from build123d import *

# Parameters (mm, degrees)
SKETCH1_W           = 69.3
SKETCH1_H           = 27
BOSS_EXTRUDE1_DEPTH = 13.2
SKETCH2_R           = 4.55
BOSS_EXTRUDE2_DEPTH = 2.25
SKETCH3_R           = 3.1
BOSS_EXTRUDE3_DEPTH = 6.25
SKETCH4_W           = 4.5
SKETCH4_H           = 12
BOSS_EXTRUDE4_DEPTH = 14


with BuildPart() as part:
    # Sketch1 → Boss-Extrude1 (new body)
    with BuildSketch(Plane.XY):
        with Locations((-34.65, 13.5)):
            Rectangle(SKETCH1_W, SKETCH1_H)
    extrude(amount=BOSS_EXTRUDE1_DEPTH)

    # Sketch2 → Boss-Extrude2 (add)
    with BuildSketch(Plane.ZY.offset(69.3)):
        with Locations((6.6, 13.5)):
            Circle(SKETCH2_R)
    extrude(amount=BOSS_EXTRUDE2_DEPTH)

    # Sketch3 → Boss-Extrude3 (add)
    with BuildSketch(Plane.ZY.offset(71.55)):
        with Locations((6.6, 13.5)):
            Circle(SKETCH3_R)
    extrude(amount=BOSS_EXTRUDE3_DEPTH)

    # Sketch4 → Boss-Extrude4 (add)
    with BuildSketch(Plane(origin=(0, 0, 0), x_dir=(0, 0, -1), z_dir=(1, 0, 0))):
        with Locations((-6.68005531, 13.414910597)):
            Rectangle(SKETCH4_W, SKETCH4_H)
    extrude(amount=BOSS_EXTRUDE4_DEPTH)


solid = part.part
Input: part model. Units: mm. Frame: model coordinates. A direction names the side the tool comes from. Coordinates: 2 decimals unless noted, no trailing zeros. Order: outer loops, then holes, each group sorted by start corner. A loop starts at its lowest first (then second) coordinate and runs counter-clockwise, first axis right, second up.
1. Cut plane A-A, the plane z = 6.6. Return loops of the section in (x, y).
Checked values:
outline: (-77.8, 10.4) - (-71.55, 10.4) - (-71.55, 8.95) - (-69.3, 8.95) - (-69.3, 0) - (0, 0) - (0, 7.41) - (14, 7.41) - (14, 19.41) - (0, 19.41) - (0, 27) - (-69.3, 27) - (-69.3, 18.05) - (-71.55, 18.05) - (-71.55, 16.6) - (-77.8, 16.6) - close
2. Access query for faces 1 (the flat face through (7, 19.415, 7)), 2 (the cylindrical face through (-70.41, 9.06, 5.61)), 3 (the flat face through (7, 7.415, 7)). Directions: +Z, -Z, +X, -X, +Y, -Y. A direction counts if a zero-diameter tool reaches every point of the face in a straight line with its end or side. Return the directions, or none.
Checked values:
face 1: +Z, -Z, +X, +Y
face 2: -X
face 3: +Z, -Z, +X, -Y
3. Cut plane B-B, the plane y = 3.5. Return loops of the section in (x, z).
Checked values:
outline: (-69.3, 0) - (0, 0) - (0, 13.2) - (-69.3, 13.2) - close
4. Contact query for flat-ended pins moving along their axis: P1, Ø1.3, axis at x = 4.5, z = 7, coming from the -Y side; P2, Ø9.5, axis at x = 6.5, y = 14.5, coming from the -Z side; P3, Ø1.3, axis at x = 8.5, z = 7.5, coming from the +Y side. Output: stop coordinate, or through.
Checked values:
P1: stops at y = 7.41
P2: stops at z = 4.43
P3: stops at y = 19.41
5. Cut plane C-C, the plane x = 1. Return loops of the section in (y, z).
Checked values:
outline: (7.41, 4.43) - (19.41, 4.43) - (19.41, 8.93) - (7.41, 8.93) - close
6. Ray query, line 1 along X through (y, z) = (2.5, 2); line 2 along X through (y, z) = (18.5, 6.5); line 3 along Y through (x, z) = (-72, 9.25). Return the intervals inside material, ascending.
Checked values:
line 1: x = -69.3 to 0
line 2: x = -69.3 to 14
line 3: y = 11.89 to 15.11
